Part model, mm, in its own coordinate system. Face numbers are marked on the shaded views. A direction names the side the tool comes from. Coordinates: 2 decimals unless noted, no trailing zeros. Write each loop counter-clockwise with the first axis right and the second up, starting at its lowest first coordinate (ties: lowest second). Pieces come first, ordered by that corner, then holes. Notation, with made-up numbers: (38, 14.25) -> (65, 14.25) arc R32 ccw to (65, 49.25) -> close; hole circle Ø5 at (26.5, 62). An arc over 180 degrees is marked (long way). Write item = value, one per line.
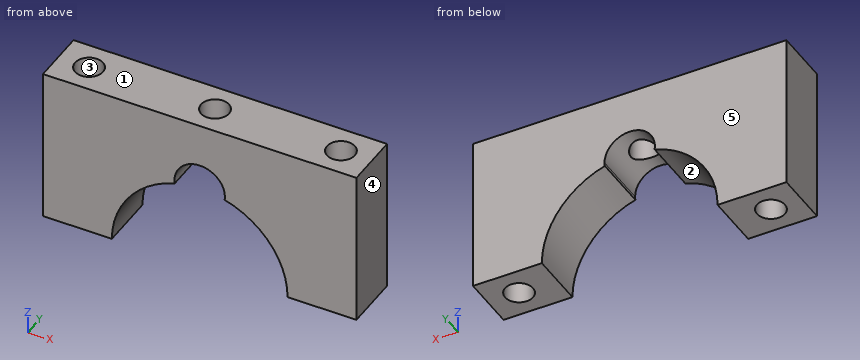
from build123d import *

# Parameters (mm, degrees)
F0_W     = 71.12
F0_H     = 35.56
F1_DEPTH = 12.7
F3_DEPTH = 12.701
F5_DEPTH = 25.4
F7_D     = 6.35
F7_DEPTH = 50.8
F7_TIP   = 1.9077324654


with BuildPart() as f1:
    # F0 (on Front) → F1 (new body)
    with BuildSketch(Plane.XZ):
        Rectangle(F0_W, F0_H)
    extrude(amount=F1_DEPTH)

    # F2 (on face) → F3 (cut, through all)
    with BuildSketch(Plane.XZ.offset(12.7)):
        with BuildLine():
            Line((-19.939, -17.78), (19.939, -17.78))
            ThreePointArc((19.939, -17.78), (0, 2.159), (-19.939, -17.78))
        make_face()
    extrude(amount=-F3_DEPTH, mode=Mode.SUBTRACT)

    # F4 (on face) → F5 (cut)
    with BuildSketch(Plane.XZ.offset(12.7)):
        with BuildLine():
            ThreePointArc((5.656007165, 1.3399713376), (5.7002327123, 1.7484247619), (5.715, 2.159))
            ThreePointArc((5.715, 2.159), (-0.4105752381, 7.8592327123), (-5.656007165, 1.3399713376))
            ThreePointArc((-5.656007165, 1.3399713376), (0, 2.159), (5.656007165, 1.3399713376))
        make_face()
    extrude(amount=-F5_DEPTH, mode=Mode.SUBTRACT)

    # F7
    with Locations(Plane.XY.offset(17.78)):
        with Locations((-28.575, -6.35), (0, -6.35), (28.575, -6.35)):
            Hole(F7_D / 2, depth=F7_DEPTH)
            with Locations((0, 0, -(F7_DEPTH + F7_TIP / 2))):  # 118° drill point
                Cone(0, F7_D / 2, F7_TIP, mode=Mode.SUBTRACT)


solid = f1.part
Q1. Saw through at A-A on x = 0. Give the cut face in (y, z) (3 decimals).
Model answer:
outline = (-12.7, 7.874) -> (-9.525, 7.874) -> (-9.525, 17.78) -> (-12.7, 17.78) -> close; (-3.175, 7.874) -> (0, 7.874) -> (0, 17.78) -> (-3.175, 17.78) -> close
Q2. Probe line 1 (X direction, y = -5.5, z = -0.5); line 2 (X direction, y = -4.5, z = -5); line 3 (Y direction, x = -29, z = -5). List the from-to ranges inside material, lowest first. Write a range as from..to.
Model answer:
line_1 = -35.56..-31.63, -25.52..-9.95, 9.95..25.52, 31.63..35.56
line_2 = -35.56..-31.16, -25.99..-15.3, 15.3..25.99, 31.16..35.56
line_3 = -12.7..-9.5, -3.2..0
Q3. Pin check, flat tip, straight feed: pin 1 (5 mm diameter, centred on x = 0, y = -6.35, fed in from +Z). Stop position of the tip, or through.
Model answer:
pin_1 = through
Q4. Mould opens along Y. For the marked faces 3, 4 and 5 say: released by +Y, released by -Y, zero draft, split by the parting line, or undercut.
Model answer:
face_3 = undercut
face_4 = zero draft
face_5 = released by +Y
Q5. Saw through at C-C on y = -6.35. Give the cut face in (x, z) (3 decimals).
Model answer:
outline = (-35.56, -17.78) -> (-31.75, -17.78) -> (-31.75, 17.78) -> (-35.56, 17.78) -> close; (-25.4, -17.78) -> (-19.939, -17.78) arc R19.939 cw to (-5.656, 1.34) arc R5.715 cw to (-3.175, 6.911) -> (-3.175, 17.78) -> (-25.4, 17.78) -> close; (3.175, 6.911) arc R5.715 cw to (5.656, 1.34) arc R19.939 cw to (19.939, -17.78) -> (25.4, -17.78) -> (25.4, 17.78) -> (3.175, 17.78) -> close; (31.75, -17.78) -> (35.56, -17.78) -> (35.56, 17.78) -> (31.75, 17.78) -> close
Q6. Which spindle directions (+Z, -Z, +X, -X, +Y, -Y) get a long thin tool onto all of the face, cutting with end or side? Do the marked faces 1 and 2. Say none if no direction does.
Model answer:
face_1 = +Z, +X, -X, +Y, -Y
face_2 = -Z, +Y, -Y
Q7. Saw through at B-B on z = -6.5. Give the cut face in (x, y) (3 decimals), and give its area (3 significant figures).
Model answer:
outline = (-35.56, -12.7) -> (-16.442, -12.7) -> (-16.442, 0) -> (-35.56, 0) -> close; (16.442, -12.7) -> (35.56, -12.7) -> (35.56, 0) -> (16.442, 0) -> close; hole circle Ø6.35 at (-28.575, -6.35); hole circle Ø6.35 at (28.575, -6.35)
area = 422 mm²
Q8. Saw through at D-D on z = 6. Give the cut face in (x, y) (3 decimals).
Model answer:
outline = (-35.56, -12.7) -> (-4.232, -12.7) -> (-4.232, 0) -> (-35.56, 0) -> close; (4.232, -12.7) -> (35.56, -12.7) -> (35.56, 0) -> (4.232, 0) -> close; hole circle Ø6.35 at (-28.575, -6.35); hole circle Ø6.35 at (28.575, -6.35)
